The listing builds one solid part. Answer for the finished solid, in the listing's coordinates (mm). A direction names the side the tool comes from. Coordinates: 2 decimals unless noted, no trailing zeros. Write each loop counter-clockwise with the first axis right and the second up, starting at its lowest first coordinate (ties: lowest second). Pieces come first, ordered by that corner, then holes. Notation, with made-up numbers: M 47.5,-3.5 L 71.5,-3.5 A23 cw 71.5,7.5 Z; hole C -0.5,-8 d3. An arc over 180 degrees is marked long. Answer as CSV lines item,"result".
```python
from build123d import *

# Parameters (mm, degrees)
F1_DEPTH = 600


with BuildPart() as f1:
    # F0 (on Top) → F1 (new body)
    with BuildSketch(Plane.XY):
        with BuildLine():
            ThreePointArc((22.454205, 15), (20.989739, 18.535534), (17.454205, 20))
            Line((17.454205, 20), (-12.545795, 20))
            ThreePointArc((-12.545795, 20), (-16.081329, 18.535534), (-17.545795, 15))
            Line((-17.545795, 15), (-17.545795, -15))
            ThreePointArc((-17.545795, -15), (-16.081329, -18.535534), (-12.545795, -20))
            Line((-12.545795, -20), (19.454205, -20))
            ThreePointArc((19.454205, -20), (21.575525, -19.12132), (22.454205, -17))
            Line((22.454205, -17), (22.454205, 15))
        make_face()
        with BuildLine():
            Line((-12.545795, 17), (17.454205, 17))
            ThreePointArc((17.454205, 17), (18.868419, 16.414214), (19.454205, 15))
            Line((19.454205, 15), (19.454205, -17))
            Line((19.454205, -17), (-12.545795, -17))
            ThreePointArc((-12.545795, -17), (-13.960009, -16.414214), (-14.545795, -15))
            Line((-14.545795, -15), (-14.545795, 15))
            ThreePointArc((-14.545795, 15), (-13.960009, 16.414214), (-12.545795, 17))
        make_face(mode=Mode.SUBTRACT)
    extrude(amount=F1_DEPTH)


solid = f1.part
```
Q1. The mould has two halves that part along Y. Classify faces 3 (the flat face through (3, 20, 296)), 4 (the flat face through (22.454, -1, 296)), 5 (the flat face through (2, 17, 296)): pulls with the +Y half, pulls with the -Y half, needs draft (parallel to the pull), parting line crosses it, or undercut.
Output:
face 3,"pulls with the +Y half"
face 4,"needs draft"
face 5,"undercut"
Q2. A flat-ended cylindrical pin translates along its axis: pin 1 Ø1 at (x, y) = (18.5, 13.5) entering from -Z. Find the tip coordinate at first contact, or state that the pin passes through.
Output:
pin 1,"through"
Q3. Straight lines are drawn through the part: line 1 (X direction, y = 4.5, z = 178.5); line 2 (Y direction, x = -7.5, z = 317); line 3 (Y direction, x = -13.5, z = 104). For each, find the intervals that lie inside material, in ascending order.
Output:
line 1,"-17.55 to -14.55, 19.45 to 22.45"
line 2,"-20 to -17, 17 to 20"
line 3,"-19.91 to -16.76, 16.76 to 19.91"
Q4. Find section C-C (z = 553). Give the vertices of the cut face in (x, y).
Output:
outline,"M -17.55,-15 A5 ccw -12.55,-20 L 19.45,-20 A3 ccw 22.45,-17 L 22.45,15 A5 ccw 17.45,20 L -12.55,20 A5 ccw -17.55,15 Z; hole M -14.55,-15 A2 ccw -12.55,-17 L 19.45,-17 L 19.45,15 A2 ccw 17.45,17 L -12.55,17 A2 ccw -14.55,15 Z"
Q5. Find section B-B (x = 11). Give the vertices of the cut face in (y, z), and give its area (3 significant figures).
Output:
outline,"M -20,0 L -17,0 L -17,600 L -20,600 Z; M 17,0 L 20,0 L 20,600 L 17,600 Z"
area,"3,600 mm2"
Q6. For faces 1 (the flat face through (2.2, -17.5, 0)), 2 (the flat face through (-14.546, 0, 296)), determine the directions among +Z, -Z, +X, -X, +Y, -Y from which every point of the face is accessible in a straight line to the end or side of a thin tool.
Output:
face 1,"-Z, +X, -X, +Y, -Y"
face 2,"+Z, -Z"
Q7. Find section A-A (y = 7.5). Give the vertices of the cut face in (x, z).
Output:
outline,"M -17.55,0 L -14.55,0 L -14.55,600 L -17.55,600 Z; M 19.45,0 L 22.45,0 L 22.45,600 L 19.45,600 Z"
